Autodesk Inventor part; units mm, degrees
ref_plane "YZ Plane" through (0, 0, 0) normal (1, 0, 0) x (0, 1, 0)
ref_plane "XZ Plane" through (0, 0, 0) normal (0, 1, 0) x (-1, 0, 0)
ref_plane "XY Plane" through (0, 0, 0) normal (0, 0, 1) x (1, 0, 0)
sketch "草圖1" plane through (0, 0, 0) normal (1, 0, 0) x (0, 1, 0)
  line L0 (-20, 30) -> (20, 30)
  line L1 (20, 30) -> (20, -30)
  line L2 (20, -30) -> (-20, -30)
  line L3 (-20, -30) -> (-20, 30)
  line L4 (-20, 30) -> (20, -30) construction
  line L5 (20, 30) -> (-20, -30) construction
  line L6 (-12.5, 20) -> (12.5, 20)
  line L7 (12.5, 20) -> (12.5, -20)
  line L8 (12.5, -20) -> (-12.5, -20)
  line L9 (-12.5, -20) -> (-12.5, 20)
  line L10 (-12.5, 20) -> (12.5, -20) construction
  line L11 (12.5, 20) -> (-12.5, -20) construction
  point P0 (0, 0)
  dimension "d0" = 40
  dimension "d1" = 60
  dimension "d2" = 25
  dimension "d3" = 40
extrude "擠出1" add sketch "草圖1" along normal blind 60
fillet "圓角1" radius 20 4 edges at (30, 20, 30) (30, -20, 30) (30, 20, -30) (30, -20, -30)
fillet "圓角2" radius 12.5 4 edges at (30, 12.5, 20) (30, -12.5, 20) (30, -12.5, -20) (30, 12.5, -20)
chamfer "倒角1" distance 5 angle 45 4 edges at (60, 14.1422, -24.1422) (60, -20, 0) (60, 14.1422, 24.1422) (60, 20, 0)
sketch "草圖2" plane through (0, -20, -10) normal (0, -1, 0) x (1, 0, 0)
  line L0 (-12, 10) -> (72, 10)
  line L1 (0, -32) -> (0, 52)
  line L2 (60, 0) -> (60, 20)
  line L3 (32, 0) -> (32, 20)
  circle A0 centre (32, 10) radius 3
  point P0 (0, 10)
  dimension "d11" = 28
  dimension "d12" = 6
extrude "擠出2" cut sketch "草圖2" against normal blind 157.75
properties part number "exercise3-8"
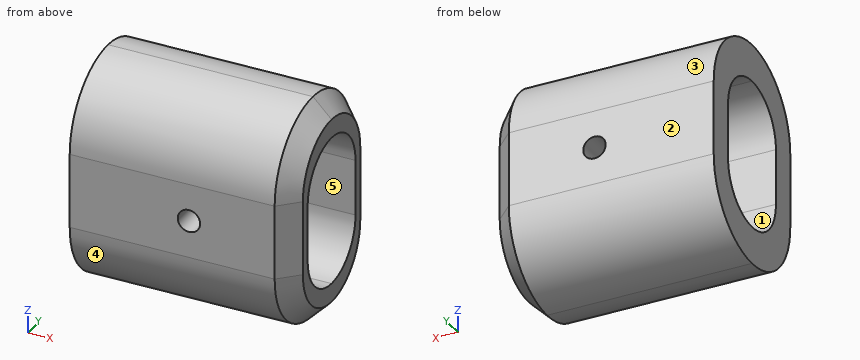
Can you work these out from the model? Positions are in its coordinate system, mm. Face numbers are marked on the shaded views. A direction names the side the tool comes from. Coordinates: 2 decimals unless noted, no trailing zeros. Loops run counter-clockwise (first coordinate to the right, second up) from the corner with the lowest first, then second, coordinate; pieces in that order, holes last.
Item 1: Suppose I cut it at B-B (z = 0). Please give me the cut outline in (x, y), then the cut area to 3 significant figures.
Answers below:
outline: (0, -20) - (29, -20) - (29, -12.5) - (0, -12.5) - close; (0, 12.5) - (29, 12.5) - (29, 20) - (0, 20) - close; (35, -20) - (55, -20) - (60, -15) - (60, -12.5) - (35, -12.5) - close; (35, 12.5) - (60, 12.5) - (60, 15) - (55, 20) - (35, 20) - close
area: 785 mm2
Item 2: Which directions (+Z, -Z, +X, -X, +Y, -Y) give clear straight access to the entire face, cutting with the end or side of a thin tool? Please do the marked faces 1 and 2.
Answers below:
face 1: +X, -X
face 2: +Z, -Z, +X, -X, +Y
Item 3: I'm going to push flat-ended pins straight in: pin 1 (3 mm diameter, centred on x = 38.5, z = 13.5, fed in from -Y); pin 2 (6 mm diameter, centred on x = 49, z = 20.5, fed in from +Y); pin 3 (5 mm diameter, centred on x = 32, z = 0, fed in from +Y); pin 4 (5 mm diameter, centred on x = 7, z = -20.5, fed in from +Y). Where does each tip first touch, or does it pass through?
Answers below:
pin 1: stops at y = -19.9
pin 2: stops at y = 18.54
pin 3: passes through
pin 4: stops at y = 18.33
Item 4: Please list where these lines run through material, in increasing order: L1, parallel to Y at x = 9.5, z = 1; L2, parallel to X at y = -14, z = 0; L3, parallel to Y at x = 20, z = 14.5.
Answers below:
L1: y = -20 to -12.5, 12.5 to 20
L2: x = 0 to 29, 35 to 60
L3: y = -19.49 to -10.36, 10.36 to 19.49
Item 5: If we mould it in two halves opening along Z, with no side actions, what happens to the marked faces 3, 4 and 5? For each: released by +Z, released by -Z, zero draft, split by the parting line, or undercut.
Answers below:
face 3: released by +Z
face 4: released by -Z
face 5: undercut
